from build123d import *

# Parameters (mm, degrees)
ESQUISSE1_R        = 3
BOSS_EXTRU_1_DEPTH = 4


with BuildPart() as part:
    # Esquisse1 → Boss.-Extru.1 (new, symmetric)
    with BuildSketch(Plane.XY):
        with BuildLine():
            Line((-4.622690842, 5.411311669), (-0.831927473, 5.942044823))
            ThreePointArc((-0.831927473, 5.942044823), (5.822154168, 1.450007187), (2.05212086, -5.638155725))
            Line((2.05212086, -5.638155725), (-8.210100717, -9.373298916))
            ThreePointArc((-8.210100717, -9.373298916), (-10.595760221, -11.203879838), (-11.5, -14.07176202))
            Line((-11.5, -14.07176202), (-11.5, -39.742063683))
            ThreePointArc((-11.5, -39.742063683), (-11.465204853, -40.330910662), (-11.361303694, -40.911562034))
            Line((-11.361303694, -40.911562034), (2.485172244, -98.46779934))
            ThreePointArc((2.485172244, -98.46779934), (3.19187279, -99.570923085), (4.429693722, -100))
            Line((4.429693722, -100), (10.429693722, -100))
            Line((10.429693722, -100), (10.429693722, -101.5))
            Line((10.429693722, -101.5), (3.279172166, -107.5))
            Line((3.279172166, -107.5), (-0.220827834, -107.5))
            ThreePointArc((-0.220827834, -107.5), (-3.315380164, -106.427307714), (-5.082131528, -103.669498351))
            Line((-5.082131528, -103.669498351), (-19.583911082, -43.389332544))
            ThreePointArc((-19.583911082, -43.389332544), (-19.89561456, -41.647378427), (-20, -39.88083749))
            Line((-20, -39.88083749), (-20, 15.11916251))
            ThreePointArc((-20, 15.11916251), (-18.966766701, 18.162969655), (-16.294095226, 19.948791641))
            Line((-16.294095226, 19.948791641), (-4.70298531, 23.054620182))
            ThreePointArc((-4.70298531, 23.054620182), (-2.756259123, 23.182215358), (-0.908890085, 22.55511807))
            Line((-0.908890085, 22.55511807), (0.649955642, 21.65511807))
            ThreePointArc((0.649955642, 21.65511807), (1.191787733, 20.347019689), (0.068498187, 19.485089305))
            Line((0.068498187, 19.485089305), (-3.931501813, 19.485089305))
            ThreePointArc((-3.931501813, 19.485089305), (-7.950786116, 17.459203239), (-8.713025593, 13.023230781))
            Line((-8.713025593, 13.023230781), (-6.812609512, 6.807249868))
            ThreePointArc((-6.812609512, 6.807249868), (-5.975040779, 5.705491773), (-4.622690842, 5.411311669))
        make_face()
        Circle(ESQUISSE1_R, mode=Mode.SUBTRACT)
    extrude(amount=BOSS_EXTRU_1_DEPTH, both=True)


solid = part.part
Geometry check sheet. Reference: the model listing, model coordinates, mm. A direction names the side the tool comes from. Coordinates: 2 decimals unless noted, no trailing zeros. Order: outer loops, then holes, each group sorted by start corner. A loop starts at its lowest first (then second) coordinate and runs counter-clockwise, first axis right, second up. Notation, with made-up numbers: (66, -7) -> (89, -7) arc R37 ccw to (89, 30) -> close; hole circle Ø7 at (19, -17.5). An arc over 180 degrees is marked (long way). Use a Markdown table: item, result. Add a question column.
1. Cross-section at B-B (z = -1). Enter the section's corners in (x, y) (1 decimal), and give its area (3 significant figures).
2. Cross-section at C-C (x = -13). Enter the section's corners in (y, z).
3. Go/stop test with flat-tipped pins: pin 1 Ø4 at (y, z) = (-29.5, 2) entering from +X; pin 2 Ø3 at (x, z) = (-8.5, -1) entering from +Y; pin 3 Ø4 at (x, z) = (-13, 2) entering from +Y; pin 4 Ø3.5 at (x, y) = (0, 0) entering from -Z. Record where each tip stops, or that it passes through.
4. Cross-section at A-A (y = 0). Enter the section's corners in (x, z).
5. Mould release check, pull along X, two halves, no side actions. Record for faces 1 (the face through (-5.992, 5.716, 0.056)), 2 (the face through (-3, 0, 0)), 3 (the face through (-19.893, -41.672, 0.056)), 4 (the face through (-7.912, 17.511, 0.056)): pulls with the +X half, pulls with the -X half, needs draft (parallel to the pull), parting line crosses it, or undercut.
6. Cross-section at D-D (y = -91.5). Enter the section's corners in (x, z), and give its area (3 significant figures).
7. Set-up check for faces 5 (the face through (-2.754, 5.673, 0.056)), 6 (the face through (-13, -37, 4)), 7 (the face through (-4.535, -69.287, 0.056)): record each of +Z, -Z, +X, -X, +Y, -Y from which the full face is reachable in a straight line by a thin tool's end or side.
8. Material ranges on L1, parallel to Y at x = 4.5, z = 2.25; L2, parallel to X at y = -29.5, z = 2; L3, parallel to Y at x = 5, z = 1.75, recorded low to high.
Filled sheet:
| question | item | result |
|---|---|---|
| 1 | outline | (-20, -39.9) arc R15 ccw to (-19.6, -43.4) -> (-5.1, -103.7) arc R5 ccw to (-0.2, -107.5) -> (3.3, -107.5) -> (10.4, -101.5) -> (10.4, -100) -> (4.4, -100) arc R2 cw to (2.5, -98.5) -> (-11.4, -40.9) arc R5 cw to (-11.5, -39.7) -> (-11.5, -14.1) arc R5 cw to (-8.2, -9.4) -> (2.1, -5.6) arc R6 ccw to (-0.8, 5.9) -> (-4.6, 5.4) arc R2 cw to (-6.8, 6.8) -> (-8.7, 13) arc R5 cw to (-3.9, 19.5) -> (0.1, 19.5) arc R1.2 ccw to (0.6, 21.7) -> (-0.9, 22.6) arc R5 ccw to (-4.7, 23.1) -> (-16.3, 19.9) arc R5 ccw to (-20, 15.1) -> close; hole circle Ø6 at (0, 0) |
| 1 | area | 1,410 mm2 |
| 2 | outline | (-70.76, -4) -> (20.83, -4) -> (20.83, 4) -> (-70.76, 4) -> close |
| 3 | pin 1 | x = -11.5 |
| 3 | pin 2 | y = 22.44 |
| 3 | pin 3 | y = 21.37 |
| 3 | pin 4 | through |
| 4 | outline | (-20, -4) -> (-3, -4) -> (-3, 4) -> (-20, 4) -> close; (3, -4) -> (6, -4) -> (6, 4) -> (3, 4) -> close |
| 5 | face 1 | undercut |
| 5 | face 2 | undercut |
| 5 | face 3 | pulls with the -X half |
| 5 | face 4 | pulls with the +X half |
| 6 | outline | (-8.01, -4) -> (0.81, -4) -> (0.81, 4) -> (-8.01, 4) -> close |
| 6 | area | 70.5 mm2 |
| 7 | face 5 | +Z, -Z |
| 7 | face 6 | +Z, +X, -X, +Y, -Y |
| 7 | face 7 | +Z, -Z, +X |
| 8 | L1 | -106.48 to -100, -3.97 to 3.97 |
| 8 | L2 | -20 to -11.5 |
| 8 | L3 | -106.06 to -100, -3.32 to 3.32 |
